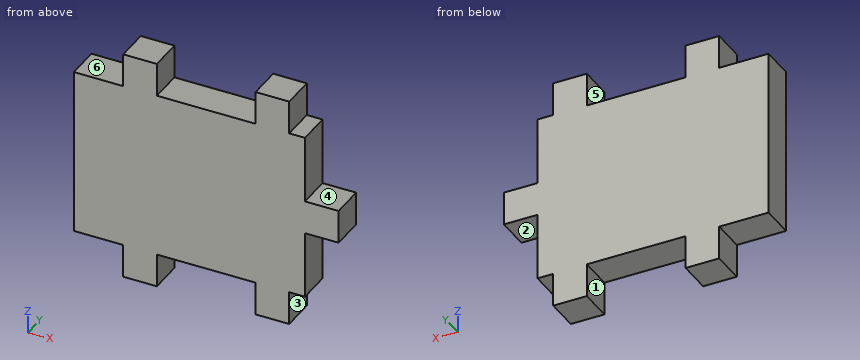
```python
from build123d import *

# Parameters (mm, degrees)
SKETCH3_W           = 87.3
SKETCH3_H           = 63.5
BOSS_EXTRUDE3_DEPTH = 12.7
SKETCH4_W           = 12.7
SKETCH4_H           = 12.7
BOSS_EXTRUDE4_DEPTH = 12.7
SKETCH5_W           = 12.7
SKETCH5_H           = 12.7
BOSS_EXTRUDE7_DEPTH = 12.7


with BuildPart() as part:
    # Sketch3 → Boss-Extrude3 (new body)
    with BuildSketch(Plane(origin=(0, 0, 0), x_dir=(1, 0, 0), z_dir=(0, 1, 0))):
        Rectangle(SKETCH3_W, SKETCH3_H)
    extrude(amount=BOSS_EXTRUDE3_DEPTH)

    # Sketch4 → Boss-Extrude4 (add)
    with BuildSketch(Plane(origin=(43.65, 0, 0), x_dir=(0, 0, -1), z_dir=(1, 0, 0))):
        with Locations((0, 6.35)):
            Rectangle(SKETCH4_W, SKETCH4_H)
    extrude(amount=BOSS_EXTRUDE4_DEPTH)

    # Sketch5 → Boss-Extrude7 (add)
    with BuildSketch(Plane.XY.offset(31.75)):
        Polygon((-12.300000038, 12.7), (-25.000000038, 12.7), (-25.000000038, 6.35), (-25.000000038, 0), (-12.300000038, 0), align=None)
        with Locations((31.349999962, 6.35)):
            Rectangle(SKETCH5_W, SKETCH5_H)
    boss_extrude7 = extrude(amount=BOSS_EXTRUDE7_DEPTH)

    # Mirror2: Boss-Extrude7 across plane
    add(boss_extrude7.mirror(Plane.XY))


solid = part.part
```
Source: CAD feature listing. Evaluate the final solid. Frame: model axes, mm. Face numbers are marked on the shaded views. A direction names the side the tool comes from. Round coordinates to 2 decimals unless told otherwise and drop trailing zeros. Write each loop counter-clockwise with the first axis right and the second up, starting at its lowest first coordinate (ties: lowest second). Pieces come first, ordered by that corner, then holes. Notation, with made-up numbers: M -34,0.25 L 2,0.25 A20 ccw 2,7.25 Z; hole C 2,2.5 d10. An arc over 180 degrees is marked long. Use CSV: the item, a comma, the result in double quotes. Start each with the question number.
Q1. Cut plane C-C on x = -4. Output: boundary loops of the cut face in (y, z), plus the area to 3 significant figures.
Q2. First-contact query: P1, Ø2, axis at x = 1.5, y = 4, coming from the -Z side; P2, Ø4, axis at y = 9, z = 41, coming from the -X side; P3, Ø2, axis at x = 27, z = 7.5, coming from the -Y side; P4, Ø4, axis at x = 8.5, y = 5.5, coming from the +Z side. Flat tips, straight axial feed; report the tip coordinate or a pass-through.
Q3. Cut plane D-D on z = 20.5. Output: boundary loops of the cut face in (x, y).
Q4. Pull-direction query (X, two-part tool) for the marked faces 1, 2 and 3; classes: +X half, -X half, draft (parallel to the pull), parting line (faces both ways), or undercut.
Q5. Access query for the marked faces 4, 5 and 6. Directions: +Z, -Z, +X, -X, +Y, -Y. A direction counts if a zero-diameter tool reaches every point of the face in a straight line with its end or side. Return the directions, or none.
Q6. Cut plane B-B on y = 7.5. Output: boundary loops of the cut face in (x, z), plus the area to 3 significant figures.
Q7. Line query: line 1 (X direction, y = 12, z = 32); line 2 (X direction, y = 8.25, z = -13); line 3 (Z direction, x = -9, y = 9.5). Output: solid intervals per line, ascending. Write a range as from..to.
Q8. Cut plane A-A on z = -36.5. Output: boundary loops of the cut face in (x, y), plus the area to 3 significant figures.
Results found:
1,outline,"M 0,-31.75 L 12.7,-31.75 L 12.7,31.75 L 0,31.75 Z"
1,area,"806 mm^2"
2,P1,"z = -31.75"
2,P2,"x = -25"
2,P3,"y = 0"
2,P4,"z = 31.75"
3,outline,"M -43.65,0 L 43.65,0 L 43.65,12.7 L -43.65,12.7 Z"
4,face 1,"undercut"
4,face 2,"draft"
4,face 3,"+X half"
5,face 4,"+Z, +X, +Y, -Y"
5,face 5,"+Z, +Y, -Y"
5,face 6,"+Z, -X, +Y, -Y"
6,outline,"M -43.65,-31.75 L -25,-31.75 L -25,-44.45 L -12.3,-44.45 L -12.3,-31.75 L 25,-31.75 L 25,-44.45 L 37.7,-44.45 L 37.7,-31.75 L 43.65,-31.75 L 43.65,-6.35 L 56.35,-6.35 L 56.35,6.35 L 43.65,6.35 L 43.65,31.75 L 37.7,31.75 L 37.7,44.45 L 25,44.45 L 25,31.75 L -12.3,31.75 L -12.3,44.45 L -25,44.45 L -25,31.75 L -43.65,31.75 Z"
6,area,"6,350 mm^2"
7,line 1,"-25..-12.3, 25..37.7"
7,line 2,"-43.65..43.65"
7,line 3,"-31.75..31.75"
8,outline,"M -25,0 L -12.3,0 L -12.3,12.7 L -25,12.7 Z; M 25,0 L 37.7,0 L 37.7,12.7 L 25,12.7 Z"
8,area,"323 mm^2"
